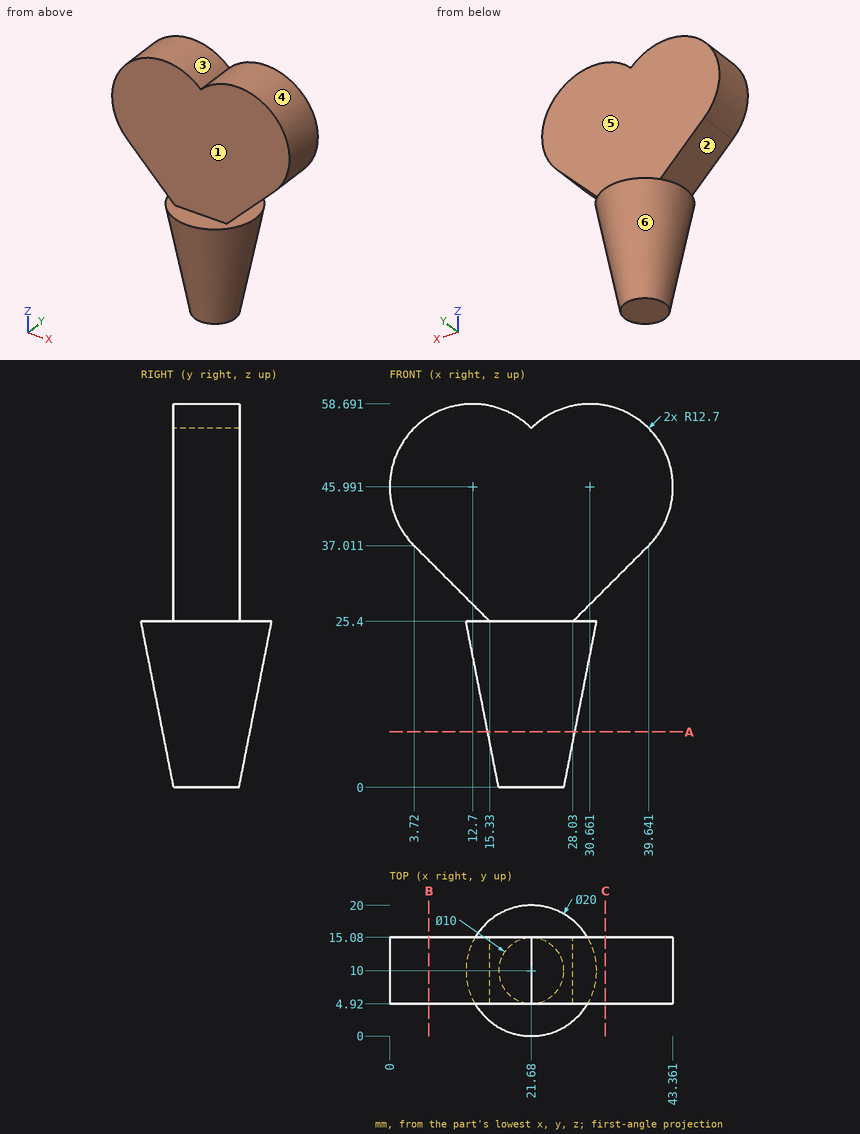
The drawing under review shows one solid part. Ordinate dimensions are in mm from its lowest x, y, z. A direction names the side the tool comes from. Round coordinates to 2 decimals unless told otherwise and drop trailing zeros. Loops run counter-clockwise (first coordinate to the right, second up) from the corner with the lowest first, then second, coordinate; pieces in that order, holes last. Notation, with made-up numbers: (68.25, 9) -> (106.25, 9) arc R15 cw to (106.25, 31) -> close; hole circle Ø11 at (61.5, 67). An arc over 180 degrees is marked (long way). One line per question, with ' | ' between items. Start each with the question number.
Item 1: Add section C-C, the plane x = 33. Write out the cut boundary in (y, z).
Item 2: Add section B-B, the plane x = 6. Write out the cut boundary in (y, z).
Item 3: Add section A-A, the plane z = 8.5. Write out the cut boundary in (x, y).
Item 4: Machinability: for the marked faces 1, 2 and 3, which of the approach directions +Z, -Z, +X, -X, +Y, -Y give a long, thin tool a straight path to every point of the face, cutting with its end or side? Answer none if there is none.
Item 5: Wall thickness on line 1 along Y through (x, z) = (33.5, 36); line 2 along X through (y, z) = (5.5, 37); line 3 along X through (y, z) = (8, 56.5) (1 decimal): over which ranges is each line inside the solid? List them lowest first. Write a range as [from, to].
Item 6: Draft analysis for pull direction X (two halves, no side actions). For the marked faces 4, 5 and 6, state which applies: +X half, -X half, draft (parallel to the pull), parting line (faces both ways), or undercut.
Item 7: For pin 1 (3 mm diameter, centred on y = 15.5, z = 30, fed in from +X); pin 2 (5 mm diameter, centred on y = 14, z = 14, fed in from -X); pin 3 (8 mm diameter, centred on x = 8.5, y = 4.5, fed in from +Z), all flat-tipped, find the tip position at first contact; note any pin that passes through.
Return value:
1) outline: (4.92, 30.37) -> (15.08, 30.37) -> (15.08, 58.47) -> (4.92, 58.47) -> close
2) outline: (4.92, 34.73) -> (15.08, 34.73) -> (15.08, 56.78) -> (4.92, 56.78) -> close
3) outline: circle Ø13.35 at (21.68, 10)
4) face 1: +Z, +X, -X, -Y | face 2: -X, +Y, -Y | face 3: +Y, -Y
5) line 1: y = [4.92, 15.08] | line 2: x = [3.73, 39.63] | line 3: x = [5.6, 19.8], [23.5, 37.8]
6) face 4: undercut | face 5: draft | face 6: parting line
7) pin 1: stops at x = 34.07 | pin 2: stops at x = 13.88 | pin 3: stops at z = 58.69
